Design review of the part built by this model. Coordinates are the model's own, in mm. A direction names the side the tool comes from. Round coordinates to 2 decimals unless told otherwise and drop trailing zeros. Loops run counter-clockwise (first coordinate to the right, second up) from the corner with the lowest first, then second, coordinate; pieces in that order, holes last. Notation, with made-up numbers: (-5.5, -7.75) -> (5.5, -7.75) arc R14 ccw to (5.5, 9.25) -> close; hole circle Ø11 at (30.25, -28.5). An arc over 180 degrees is marked (long way). Use a Markdown table: item, result. Add a question column.
from build123d import *

# Parameters (mm, degrees)
F1_DEPTH = 812.8
F2_R     = 2.6162
F3_DEPTH = 3.176
F4_R     = 2.6162
F5_DEPTH = 3.176


with BuildPart() as f1:
    # F0 (on Front) → F1 (new body)
    with BuildSketch(Plane.XZ):
        with BuildLine():
            Line((-25.4, 0), (0, 0))
            ThreePointArc((0, 0), (-0.929936, 2.245064), (-3.175, 3.175))
            Line((-3.175, 3.175), (-19.05, 3.175))
            ThreePointArc((-19.05, 3.175), (-21.295064, 4.104936), (-22.225, 6.35))
            Line((-22.225, 6.35), (-22.225, 22.225))
            ThreePointArc((-22.225, 22.225), (-23.154936, 24.470064), (-25.4, 25.4))
            Line((-25.4, 25.4), (-25.4, 0))
        make_face()
    extrude(amount=F1_DEPTH)

    # F2 (on face) → F3 (cut, through all)
    with BuildSketch(Plane.YZ.offset(-22.225)):
        with Locations((-558.8, 14.2875)):
            Circle(F2_R)
        with Locations((-406.4, 14.2875)):
            Circle(F2_R)
        with Locations((-254, 14.2875)):
            Circle(F2_R)
    extrude(amount=-F3_DEPTH, mode=Mode.SUBTRACT)

    # F4 (on face) → F5 (cut, through all)
    with BuildSketch(Plane.XY.offset(3.175)):
        with Locations((-11.1125, -804.8625)):
            Circle(F4_R)
        with Locations((-11.1125, -7.9375)):
            Circle(F4_R)
    extrude(amount=-F5_DEPTH, mode=Mode.SUBTRACT)


solid = f1.part
1. Insertion check: P1, Ø3, axis at y = -232.5, z = 22, coming from the +X side (3 decimals); P2, Ø12.5, axis at x = -9.5, y = -293.5, coming from the +Z side (3 decimals). Each pin has a flat end and moves straight along its axis. Give the tip position at first contact, or say it passes through.
2. Consider section A-A on y = -187. State the section outline as (x, z) points (3 decimals).
3. To check wall thickness, follow probe 1 along Z at (x, y) = (-24.6, -254); probe 2 along X at (y, z) = (-228.5, 20) (3 decimals); probe 3 along Z at (x, y) = (-8.5, -255.5) (3 decimals). State the ranges of each line that lie inside material, in increasing order. Write a range as from..to.
4. For faces 1 (the face through (-11, -401, 3.175)), 2 (the face through (-22.2, 0, 5.2)), list the 3-axis set-ups (+Z, -Z, +X, -X, +Y, -Y) from which the entire face can be reached by the end or side of a thin tool; tool diameter is ignored.
Verdict:
| question | item | result |
|---|---|---|
| 1 | P1 | stops at x = -22.225 |
| 1 | P2 | stops at z = 3.175 |
| 2 | outline | (-25.4, 0) -> (0, 0) arc R3.175 ccw to (-3.175, 3.175) -> (-19.05, 3.175) arc R3.175 cw to (-22.225, 6.35) -> (-22.225, 22.225) arc R3.175 ccw to (-25.4, 25.4) -> close |
| 3 | probe 1 | z = 0..11.67, 16.9..25.3 |
| 3 | probe 2 | x = -25.4..-22.225 |
| 3 | probe 3 | z = 0..3.175 |
| 4 | face 1 | +Z, +X, +Y, -Y |
| 4 | face 2 | +Z, -Z, +X, -X, +Y |
